```python
from build123d import *

# Parameters (mm, degrees)
F0_W     = 50.8
F0_H     = 12.7
F1_DEPTH = 25.4
F2_W     = 12.7
F2_H     = 6.35
F3_DEPTH = 25.4
F4_R     = 6.35
F4_R_2   = 6.420699
F5_DEPTH = 25.4


with BuildPart() as f1:
    # F0 (on Front) → F1 (new body)
    with BuildSketch(Plane.XZ):
        Polygon((-62.537882, 44.45), (-62.537882, 0), (-49.837882, 0), (-49.837882, 12.7), (-49.837882, 44.45), align=None)
        with Locations((-24.437882, 6.35)):
            Rectangle(F0_W, F0_H)
    extrude(amount=F1_DEPTH)

    # F2 (on face) → F3 (cut)
    with BuildSketch(Plane.YZ.offset(-49.837882)):
        with Locations((-12.7, 41.275)):
            Rectangle(F2_W, F2_H)
        with BuildLine():
            Line((-6.35, 38.1), (-19.05, 38.1))
            ThreePointArc((-19.05, 38.1), (-12.7, 31.75), (-6.35, 38.1))
        make_face()
    extrude(amount=-F3_DEPTH, mode=Mode.SUBTRACT)

    # F4 (on face) → F5 (cut)
    with BuildSketch(Plane.XY.offset(12.7)):
        with Locations((-37.137882, -13.766274)):
            Circle(F4_R)
        with Locations((-11.737882, -13.559262)):
            Circle(F4_R_2)
        with BuildLine():
            ThreePointArc((-6.927767, 0), (0.847206, -12.576641), (-6.513743, -25.4))
            Line((-6.513743, -25.4), (0.962118, -25.4))
            Line((0.962118, -25.4), (0.962118, 0))
            Line((0.962118, 0), (-6.927767, 0))
        make_face()
    extrude(amount=-F5_DEPTH, mode=Mode.SUBTRACT)


solid = f1.part
```
Verification items for the finished model (mm, model axes). A direction names the side the tool comes from. Coordinates: 2 decimals unless noted, no trailing zeros. Write each loop counter-clockwise with the first axis right and the second up, starting at its lowest first coordinate (ties: lowest second). Pieces come first, ordered by that corner, then holes. Notation, with made-up numbers: (-15.75, 89) - (5.25, 89) arc R20 cw to (5.25, 111) - close; hole circle Ø5 at (-4, -10.75). An arc over 180 degrees is marked (long way). One line per question, with ' | ' between items. Start each with the question number.
1. Material ranges on line 1 along X through (y, z) = (-10, 10); line 2 along X through (y, z) = (-17, 6); line 3 along Y through (x, z) = (-59, 38), recorded low to high.
2. Section check D-D (x = -37). Enter the section's corners in (y, z).
3. Section check C-C (z = 36.5). Enter the section's corners in (x, y), plus the area to 3 significant figures.
4. Access from +Z, -Z, +X, -X, +Y, -Y to the whole of each face (thin tool, end or side, straight path). Record for faces 1 (the flat face through (-25, -13, 12.7)), 2 (the flat face through (-56, -6.35, 41)), 3 (the cylindrical face through (0.842, -12.359, 6.439)).
5. Section check A-A (x = -54). Enter the section's corners in (y, z), plus the area to 3 significant figures.
6. Section check B-B (y = -18). Enter the section's corners in (x, z).
7. Draft check along X on faces 4 (the flat face through (-56, -22, 44.45)), 5 (the flat face through (-49.838, -13, 25)), 6 (the cylindrical face through (-41.818, -9.475, 6.439)), 7 (the cylindrical face through (-5.614, -11.631, 6.439)). Enter one of: released by +X, released by -X, zero draft, split by the parting line, or undercut.
8. Gauge pin test, flat ends, axial feed: P1, Ø3, axis at x = -11.5, y = -6.5, coming from the +Z side; P2, Ø1, axis at x = -34, z = 9.5, coming from the +Y side; P3, Ø7.5, axis at y = -11.5, z = 21, coming from the +X side. Record the tip position at first contact, or that the pin passes through.
Computed values:
1) line 1: -62.54 to -42.25, -32.03 to -17.08, -6.39 to 0.57 | line 2: -62.54 to -42.6, -31.67 to -17.16, -6.32 to 0.23 | line 3: -25.4 to -19.05, -6.35 to 0
2) outline: (-25.4, 0) - (-20.11, 0) - (-20.11, 12.7) - (-25.4, 12.7) - close; (-7.42, 0) - (0, 0) - (0, 12.7) - (-7.42, 12.7) - close
3) outline: (-62.54, -25.4) - (-49.84, -25.4) - (-49.84, -18.85) - (-62.54, -18.85) - close; (-62.54, -6.55) - (-49.84, -6.55) - (-49.84, 0) - (-62.54, 0) - close | area: 166 mm²
4) face 1: +Z, +X, +Y, -Y | face 2: +Z, +X, -X | face 3: +Z, -Z, +X
5) outline: (-25.4, 0) - (0, 0) - (0, 44.45) - (-6.35, 44.45) - (-6.35, 38.1) arc R6.35 cw to (-19.05, 38.1) - (-19.05, 44.45) - (-25.4, 44.45) - close | area: 985 mm²
6) outline: (-62.54, 0) - (-41.87, 0) - (-41.87, 12.7) - (-49.84, 12.7) - (-49.84, 34.6) - (-62.54, 34.6) - close; (-32.41, 0) - (-16.38, 0) - (-16.38, 12.7) - (-32.41, 12.7) - close; (-7.1, 0) - (-0.11, 0) - (-0.11, 12.7) - (-7.1, 12.7) - close
7) face 4: zero draft | face 5: released by +X | face 6: undercut | face 7: undercut
8) P1: z = 12.7 | P2: y = 0 | P3: x = -49.84
